The listing builds one solid part. Answer for the finished solid, in the listing's coordinates (mm). Give positions to 0.01 mm unless a question says otherwise; leave off trailing zeros. Write each loop counter-clockwise with the first axis right and the second up, starting at its lowest first coordinate (ties: lowest second). Pieces come first, ordered by that corner, then holes. Notation, with made-up numbers: (8.5, -24.75) - (66.5, -24.75) arc R16 cw to (66.5, 5.25) - close; hole circle Ø5 at (68.25, 14.5). An arc over 180 degrees is marked (long way). Return JSON: item names as keys, results as strings.
from build123d import *

# Parameters (mm, degrees)
F1_DEPTH = 12.7
F3_D     = 19.05
F5_D     = 6.35
F7_D     = 3.96748


with BuildPart() as f1:
    # F0 (on Front) → F1 (new body)
    with BuildSketch(Plane.XZ):
        with BuildLine():
            Line((711.2, 25.4), (736.6, 0))
            Line((736.6, 0), (1447.8, 0))
            Line((1447.8, 0), (1473.2, 25.4))
            Line((1473.2, 25.4), (1473.2, 537.3624))
            Line((1473.2, 537.3624), (1447.8, 562.7624))
            Line((1447.8, 562.7624), (736.6, 562.7624))
            Line((736.6, 562.7624), (711.2, 537.3624))
            Line((711.2, 537.3624), (711.2, 472.8718))
            ThreePointArc((711.2, 472.8718), (696.321024, 436.950776), (660.4, 422.0718))
            Line((660.4, 422.0718), (25.4, 422.0718))
            Line((25.4, 422.0718), (0, 396.6718))
            Line((0, 396.6718), (0, 166.0906))
            Line((0, 166.0906), (25.4, 140.6906))
            Line((25.4, 140.6906), (660.4, 140.6906))
            ThreePointArc((660.4, 140.6906), (696.321024, 125.811624), (711.2, 89.8906))
            Line((711.2, 89.8906), (711.2, 25.4))
        make_face()
    extrude(amount=F1_DEPTH)

    # F3 (through all)
    with Locations(Plane.XZ.offset(12.7)):
        with Locations((1138.202135, 363.479406), (1138.202135, 205.5876), (1390.193105, 205.5876), (1390.193105, 363.479406)):
            Hole(F3_D / 2)

    # F5 (through all)
    with Locations(Plane.XZ.offset(12.7)):
        with Locations((1435.1, 396.862477), (1460.5, 396.862477), (1435.1, 205.5876), (1460.5, 205.5876)):
            Hole(F5_D / 2)

    # F7 (through all)
    with Locations(Plane.XZ.offset(12.7)):
        with Locations((743.7374, 536.535431), (743.7374, 511.135431), (786.6126, 511.135431), (786.6126, 536.535431), (743.7374, 26.226969), (743.7374, 51.626969), (786.6126, 51.626969), (786.6126, 26.226969), (1397.7874, 26.226969), (1397.7874, 51.626969), (1440.6626, 26.226969), (1440.6626, 51.626969), (1397.7874, 511.135431), (1397.7874, 536.535431), (1440.6626, 536.535431), (1440.6626, 511.135431)):
            Hole(F7_D / 2)


solid = f1.part
Item 1: Consider L1, parallel to X at y = -2, z = 51.5; L2, parallel to Z at x = 657, y = -0.25; L3, parallel to X at y = -3, z = 486.5. Determine where each line is inside the solid, lowest interval first.
Answer below:
{"L1": "x = 711.2 to 741.76, 745.72 to 784.63, 788.59 to 1395.81, 1399.77 to 1438.68, 1442.64 to 1473.2", "L2": "z = 140.69 to 422.07", "L3": "x = 711.2 to 1473.2"}
Item 2: A cutting plane is placed at A-A on x = 439.5. Determine the outline of the cut face in (y, z), then the cut area to 3 significant figures.
Answer below:
{"outline": "(-12.7, 140.69) - (0, 140.69) - (0, 422.07) - (-12.7, 422.07) - close", "area": "3,570 mm²"}
Item 3: A cutting plane is placed at B-B on y = -3.25. Give the number of separate pieces and of enclosed holes in the cut face, then the cut area to 3 significant figures.
Answer below:
{"separate pieces": "1", "enclosed holes": "24", "area": "627,000 mm²"}
Item 4: Flat-ended cylindrical pins translate along their axes: P1, Ø5, axis at x = 1440.66, z = 511.14, coming from the +Y side; P2, Ø6.5, axis at x = 347, y = -7.5, coming from the -Z side; P3, Ø4, axis at x = 486.5, y = -8.5, coming from the +Z side. Find the tip coordinate at first contact, or state that the pin passes through.
Answer below:
{"P1": "stops at y = 0", "P2": "stops at z = 140.69", "P3": "stops at z = 422.07"}
